Part model, mm, in its own coordinate system. Face numbers are marked on the shaded views. A direction names the side the tool comes from. Give positions to 0.01 mm unless a question says otherwise; leave off trailing zeros. Order: outer loops, then holes, each group sorted by start corner. A loop starts at its lowest first (then second) coordinate and runs counter-clockwise, first axis right, second up.
1. Slice it at B-B on y = -12.75. List the corners of the cut face in (x, z) (1 decimal).
2. Slice it at D-D on x = 174.5. List the corners of the cut face in (y, z) (1 decimal).
3. Mould opens along Z. For the marked faces 3, 4, 5 and 6 say: +Z half, -Z half, draft (parallel to the pull), parting line (faces both ways), or undercut.
4. Slice it at C-C on z = 12.7. List the corners of the cut face in (x, y) (3 decimals), and give its area (3 significant figures).
5. Drop flat-ended pins along their axis: pin 1 Ø4 at (x, y) = (32.5, -5.5) entering from -Z; pin 2 Ø10 at (x, z) = (33, 81) entering from +Y; pin 3 Ø7.5 at (y, z) = (-12, 14.5) entering from +X (3 decimals); pin 4 Ø1.5 at (y, z) = (-18, 91) entering from +X. Give the stop position or say it passes through.
6. Which spindle directions (+Z, -Z, +X, -X, +Y, -Y) get a long thin tool onto all of the face, cutting with end or side? Do the marked faces 1 and 2. Say none if no direction does.
7. Slice it at A-A on x = 56. List the corners of the cut face in (y, z) (1 decimal), and give its area (3 significant figures).
8. Probe line 1 (Z direction, x = 35, y = -8) (1 decimal); line 2 (Z direction, x = 24, y = -17.75) (1 decimal); line 3 (Z direction, x = 69, y = -22.75). List the from-to ranges inside material, lowest first.
from build123d import *

# Parameters (mm, degrees)
F1_DEPTH = 25.4
F2_T     = -3.175
F3_R     = 3.96875
F4_DEPTH = 25.4


with BuildPart() as f1:
    # F0 (on Front) → F1 (new body)
    with BuildSketch(Plane.XZ):
        Polygon((0, 182.5625), (0, 0), (111.125, 0), (111.125, 25.4), (25.4, 25.4), (25.4, 157.1625), (190.5, 157.1625), (190.5, 182.5625), align=None)
    extrude(amount=F1_DEPTH)

    # F2
    f2_openings = [f1.faces().sort_by_distance(p)[0] for p in [
        (190.5, -12.7, 169.8625),
        (111.125, -12.7, 12.7),
    ]]
    offset(amount=F2_T, openings=f2_openings, kind=Kind.INTERSECTION)

    # F3 (on face) → F4 (cut)
    with BuildSketch(Plane.XZ.offset(25.4)):
        with Locations((98.425, 12.7)):
            Circle(F3_R)
    extrude(amount=-F4_DEPTH, mode=Mode.SUBTRACT)


solid = f1.part
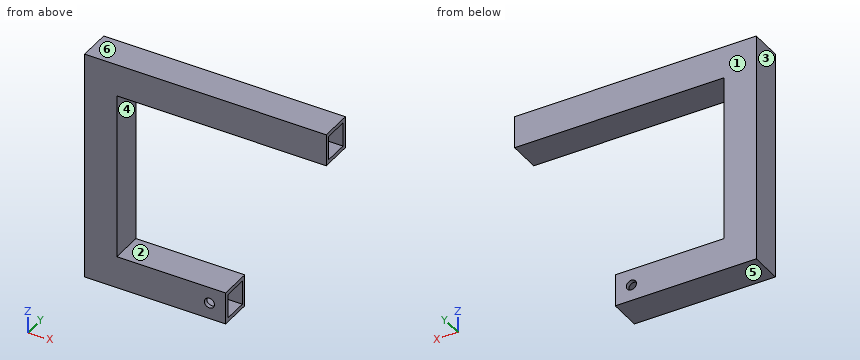
Data:
1. outline: (0, 0) - (111.1, 0) - (111.1, 3.2) - (3.2, 3.2) - (3.2, 179.4) - (190.5, 179.4) - (190.5, 182.6) - (0, 182.6) - close; (22.2, 22.2) - (111.1, 22.2) - (111.1, 25.4) - (25.4, 25.4) - (25.4, 157.2) - (190.5, 157.2) - (190.5, 160.3) - (22.2, 160.3) - close
2. outline: (-25.4, 157.2) - (0, 157.2) - (0, 182.6) - (-25.4, 182.6) - close; hole (-22.2, 160.3) - (-3.2, 160.3) - (-3.2, 179.4) - (-22.2, 179.4) - close
3. face 3: draft
3. face 4: undercut
3. face 5: -Z half
3. face 6: +Z half
4. outline: (0, -25.4) - (94.456, -25.4) - (94.456, -22.225) - (3.175, -22.225) - (3.175, -3.175) - (94.456, -3.175) - (94.456, 0) - (0, 0) - close; (102.394, -25.4) - (111.125, -25.4) - (111.125, -22.225) - (102.394, -22.225) - close; (102.394, -3.175) - (111.125, -3.175) - (111.125, 0) - (102.394, 0) - close
4. area: 716 mm2
5. pin 1: stops at z = 0
5. pin 2: passes through
5. pin 3: stops at x = 3.175
5. pin 4: stops at x = 25.4
6. face 1: +Z, -Z, +X, -X, +Y
6. face 2: +X, +Y, -Y
7. outline: (-25.4, 0) - (0, 0) - (0, 25.4) - (-25.4, 25.4) - close; (-25.4, 157.2) - (0, 157.2) - (0, 182.6) - (-25.4, 182.6) - close; hole (-22.2, 3.2) - (-3.2, 3.2) - (-3.2, 22.2) - (-22.2, 22.2) - close; hole (-22.2, 160.3) - (-3.2, 160.3) - (-3.2, 179.4) - (-22.2, 179.4) - close
7. area: 565 mm2
8. line 1: z = 0 to 3.2, 22.2 to 25.4, 157.2 to 160.3, 179.4 to 182.6
8. line 2: z = 0 to 3.2, 22.2 to 160.3, 179.4 to 182.6
8. line 3: z = 0 to 25.4, 157.16 to 182.56
